Build history of the part. All positions in model axes, mm. Face numbers are marked on the shaded views. A direction names the side the tool comes from. Round coordinates to 2 decimals unless told otherwise and drop trailing zeros. Loops run counter-clockwise (first coordinate to the right, second up) from the corner with the lowest first, then second, coordinate; pieces in that order, holes last. Notation, with made-up numbers: (86.5, 23) - (94.5, 23) arc R22 ccw to (94.5, 60) - close; hole circle Ø5 at (54.25, -6). An arc over 180 degrees is marked (long way). Use one line per item in the form item = value. Start each with the question number.
Q1. Drill centre lines: line 1 (Z direction, x = -4.35, y = 5.25); line 2 (Z direction, x = -1.1, y = -9.5); line 3 (Y direction, x = -1.85, z = 20.5). Where is each one in solid material? Low to high.
Q2. Saw through at D-D (y = -3.75). Give the cut face in (x, z).
Q3. Mould opens along Z. For the marked faces 1, 2 and 3 say: released by +Z, released by -Z, zero draft, split by the parting line, or undercut.
Q4. Saw through at C-C (z = 19). Give the cut face in (x, y), then the cut area to 3 significant figures.
Q5. Saw through at A-A (y = 5.75). Give the cut face in (x, z).
Q6. 3-axis set-ups, long thin cutter, end or side, ignore diameter. For the marked faces 4, 5 and 6: which of +Z, -Z, +X, -X, +Y, -Y reach the whole face in a straight line?
Q7. Saw through at B-B (x = -0.8). Give the cut face in (y, z), then the cut area to 3 significant figures.
Q8. Pin check, flat tips, straight feed: pin 1 (3 mm diameter, centred on x = -2, z = -1, fed in from +Y); pin 2 (1.4 mm diameter, centred on y = -19, z = -17.5, fed in from -X); pin 3 (1.4 mm diameter, centred on x = -1, z = 12, fed in from +Y). Stop position of each tip, or through.
```python
from build123d import *

# Parameters (mm, degrees)
BOSS_EXTRUDE2_DEPTH      = 6
BOSS_EXTRUDE3_DEPTH      = 18.469887
BOSS_EXTRUDE3_DEPTH_BACK = 31.530113


with BuildPart() as part:
    # Sketch1 → Boss-Extrude2 (new body)
    with BuildSketch(Plane(origin=(0, 0, 0), x_dir=(0, 0, -1), z_dir=(1, 0, 0))):
        Polygon((-3.1, 0), (-3.1, 10), (-6.530112864, 10), (-6.530112864, -20), (6.530112864, -20), (6.530112864, 10), (3.1, 10), (3.1, 0), align=None)
    extrude(amount=-BOSS_EXTRUDE2_DEPTH)

    # Sketch2 → Boss-Extrude3 (add, two sides: drawn at the far end of the back side and taken through both)
    with BuildSketch(Plane.XY.offset(6.530112864).offset(-BOSS_EXTRUDE3_DEPTH_BACK)):
        with BuildLine():
            Line((0, -20), (-5.707191464, -20))
            Line((-5.707191464, -20), (-5.707191464, -18.292808536))
            ThreePointArc((-5.707191464, -18.292808536), (-4.535618589, -15.464381411), (-1.707191464, -14.292808536))
            Line((-1.707191464, -14.292808536), (0, -14.292808536))
            Line((0, -14.292808536), (0, -20))
        make_face()
    extrude(amount=BOSS_EXTRUDE3_DEPTH + BOSS_EXTRUDE3_DEPTH_BACK)


solid = part.part
```
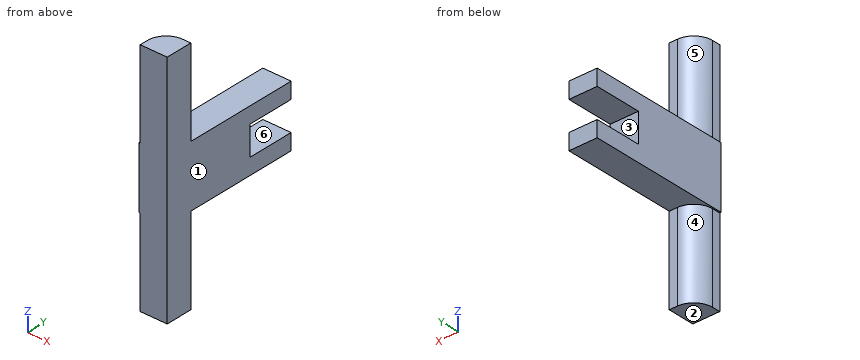
Report:
q1.line_1 = -6.53 to -3.1, 3.1 to 6.53
q1.line_2 = -6.53 to 6.53
q1.line_3 = -20 to -14.3
q2.outline = (-6, -6.53) - (0, -6.53) - (0, 6.53) - (-6, 6.53) - close
q3.face_1 = zero draft
q3.face_2 = released by -Z
q3.face_3 = undercut
q4.outline = (-5.71, -20) - (0, -20) - (0, -14.29) - (-1.71, -14.29) arc R4 ccw to (-5.71, -18.29) - close
q4.area = 29.1 mm²
q5.outline = (-6, -6.53) - (0, -6.53) - (0, -3.1) - (-6, -3.1) - close; (-6, 3.1) - (0, 3.1) - (0, 6.53) - (-6, 6.53) - close
q6.face_4 = -Z, -X, +Y
q6.face_5 = +Z, -X, +Y
q6.face_6 = +X, -X, +Y
q7.outline = (-20, -25) - (-14.29, -25) - (-14.29, -6.53) - (10, -6.53) - (10, -3.1) - (0, -3.1) - (0, 3.1) - (10, 3.1) - (10, 6.53) - (-14.29, 6.53) - (-14.29, 25) - (-20, 25) - close
q7.area = 541 mm²
q8.pin_1 = 0
q8.pin_2 = -5.71
q8.pin_3 = -14.29
